Could you check a few things on this model? Use its own coordinates, in mm. Coordinates: 2 decimals unless noted, no trailing zeros. Write each loop counter-clockwise with the first axis right and the second up, starting at its lowest first coordinate (ties: lowest second). Pieces come first, ordered by that corner, then holes. Notation, with made-up numbers: M 58,71 L 114,71 A17 cw 114,90 Z; hole C 52,4.5 d1. An arc over 180 degrees is marked long. Write item = value, one per line.
```python
from build123d import *

# Parameters (mm, degrees)
SKETCH_1_W          = 130
SKETCH_1_H          = 95
EXTRUDE_1_DEPTH     = 3
SKETCH_3_R          = 1.5
CUT_EXTRUDE_2_DEPTH = 10
SKETCH_4_R          = 1.5
CUT_EXTRUDE_3_DEPTH = 10
SKETCH_5_R          = 7.5
CUT_EXTRUDE_4_DEPTH = 10


with BuildPart() as part:
    # 草图1 → 凸台-拉伸1 (new body)
    with BuildSketch(Plane.XY):
        Rectangle(SKETCH_1_W, SKETCH_1_H)
    extrude(amount=EXTRUDE_1_DEPTH)

    # 草图3 → 切除-拉伸2 (cut)
    with BuildSketch(Plane(origin=(0, 0, 0), x_dir=(-1, 0, 0), z_dir=(0, 0, -1))):
        with Locations((-57.767112616, -26.5)):
            Circle(SKETCH_3_R)
        with Locations((-41.767112616, -26.5)):
            Circle(SKETCH_3_R)
        with Locations((42.232887384, -26.5)):
            Circle(SKETCH_3_R)
        with Locations((58.232887384, -26.5)):
            Circle(SKETCH_3_R)
    extrude(amount=-CUT_EXTRUDE_2_DEPTH, mode=Mode.SUBTRACT)

    # 草图4 → 切除-拉伸3 (cut)
    with BuildSketch(Plane(origin=(0, 0, 0), x_dir=(-1, 0, 0), z_dir=(0, 0, -1))):
        with Locations((-46.767112616, 42.5)):
            Circle(SKETCH_4_R)
        with Locations((-46.767112616, 22.5)):
            Circle(SKETCH_4_R)
        with Locations((47.232887384, 42.5)):
            Circle(SKETCH_4_R)
        with Locations((47.232887384, 22.5)):
            Circle(SKETCH_4_R)
    extrude(amount=-CUT_EXTRUDE_3_DEPTH, mode=Mode.SUBTRACT)

    # 草图5 → 切除-拉伸4 (cut)
    with BuildSketch(Plane.XY.offset(3)):
        with Locations((0, 7.452587902)):
            Circle(SKETCH_5_R)
    extrude(amount=-CUT_EXTRUDE_4_DEPTH, mode=Mode.SUBTRACT)


solid = part.part
```
Item 1: Imagine slicing it at A-A (y = 42.5). Write out the boundary of the cut face in (x, z), and give its area (3 significant figures).
Numbers:
outline = M -65,0 L -48.73,0 L -48.73,3 L -65,3 Z; M -45.73,0 L 45.27,0 L 45.27,3 L -45.73,3 Z; M 48.27,0 L 65,0 L 65,3 L 48.27,3 Z
area = 372 mm²
Item 2: Imagine slicing it at C-C (x = 0). Write out the boundary of the cut face in (y, z).
Numbers:
outline = M -47.5,0 L -0.05,0 L -0.05,3 L -47.5,3 Z; M 14.95,0 L 47.5,0 L 47.5,3 L 14.95,3 Z
Item 3: If we mould it in two halves opening along Y, with no side actions, what happens to faces 1 (the face through (-48.62, 41.93, 1.48)), 2 (the face through (-1, 47.5, 1)), 3 (the face through (65, -1, 1)), 4 (the face through (-48.664, 22.951, 1.479))? For each: pulls with the +Y half, pulls with the -Y half, needs draft (parallel to the pull), parting line crosses it, or undercut.
Numbers:
face_1 = undercut
face_2 = pulls with the +Y half
face_3 = needs draft
face_4 = undercut
Item 4: Imagine slicing it at D-D (z = 2.4). State how many separate pieces and enclosed holes the cut face has, and give its area (3 significant figures).
Numbers:
separate_pieces = 1
enclosed_holes = 9
area = 12,100 mm²
Item 5: If I drill on line 1 along X through (y, z) = (23, 2.55); line 2 along Y through (x, z) = (-42.5, 1.6); line 3 along X through (y, z) = (-26, 0.8), over which ranges is the centre line in solid material (lowest first)?
Numbers:
line_1 = -65 to -48.65, -45.82 to 45.35, 48.18 to 65
line_2 = -47.5 to -27.98, -25.02 to 47.5
line_3 = -65 to -59.65, -56.82 to -43.65, -40.82 to 40.35, 43.18 to 56.35, 59.18 to 65
Item 6: Imagine slicing it at B-B (y = -26.5). Write out the boundary of the cut face in (x, z), and give its area (3 significant figures).
Numbers:
outline = M -65,0 L -59.73,0 L -59.73,3 L -65,3 Z; M -56.73,0 L -43.73,0 L -43.73,3 L -56.73,3 Z; M -40.73,0 L 40.27,0 L 40.27,3 L -40.73,3 Z; M 43.27,0 L 56.27,0 L 56.27,3 L 43.27,3 Z; M 59.27,0 L 65,0 L 65,3 L 59.27,3 Z
area = 354 mm²
